```python
from build123d import *

# Parameters (mm, degrees)
BOSS_EXTRUDE1_DEPTH      = 49
BOSS_EXTRUDE1_DEPTH_BACK = 49
BOSS_EXTRUDE2_DEPTH      = 5
BOSS_EXTRUDE4_DEPTH      = 15
BOSS_EXTRUDE5_DEPTH      = 22
BOSS_EXTRUDE5_DEPTH_BACK = 22
BOSS_EXTRUDE6_REACH      = 127.363
SKETCH7_R                = 1.75
CUT_EXTRUDE1_DEPTH       = 25
SKETCH8_R                = 2.75
CUT_EXTRUDE2_DEPTH       = 25
FILLET1_R                = 10
FILLET2_R                = 3
SKETCH9_W                = 3
SKETCH9_H                = 102
BOSS_EXTRUDE7_DEPTH      = 25


with BuildPart() as part:
    # Sketch1 → Boss-Extrude1 (new, two sides: drawn at the far end of the back side and taken through both)
    with BuildSketch(Plane.XY.offset(-BOSS_EXTRUDE1_DEPTH_BACK)):
        Polygon((0, 0), (50, 40), (50, 20.790627288), (9.370425713, -11.713032142), (13.118595999, -16.398244998), (56, 17.906878203), (56, 52.483749085), (-3.748170285, 4.685212857), align=None)
    extrude(amount=BOSS_EXTRUDE1_DEPTH + BOSS_EXTRUDE1_DEPTH_BACK)

    # Sketch2 → Boss-Extrude2 (add)
    with BuildSketch(Plane.XY.offset(49)):
        Polygon((-3.748170285, 4.685212857), (13.118595999, -16.398244998), (56, 17.906878203), (56, 52.483749085), align=None)
    boss_extrude2 = extrude(amount=BOSS_EXTRUDE2_DEPTH)

    # Mirror1: Boss-Extrude2 across plane
    add(boss_extrude2.mirror(Plane.XY))

    # Sketch4 → Boss-Extrude4 (add)
    with BuildSketch(Plane(origin=(9.370425713, -11.713032142, 0), x_dir=(0.7808688094430303, 0.6246950475544244, 0), z_dir=(-0.6246950475544244, 0.7808688094430304, 0))):
        Polygon((52.031242374, 49), (0, 49), (52.031242374, 44), align=None)
        Polygon((52.031242374, -49), (52.031242374, -44), (0, -49), align=None)
    extrude(amount=BOSS_EXTRUDE4_DEPTH)

    # Sketch5 → Boss-Extrude5 (add, two sides: drawn at the far end of the back side and taken through both)
    with BuildSketch(Plane(origin=(56, 0, 0), x_dir=(0, 0, -1), z_dir=(1, 0, 0)).offset(-BOSS_EXTRUDE5_DEPTH_BACK)):
        with BuildLine():
            Line((-49, 101.483749085), (-59, 101.483749085))
            Line((-59, 101.483749085), (-59, 98.483749085))
            Line((-59, 98.483749085), (-51.91338941, 98.483749085))
            ThreePointArc((-51.91338941, 98.483749085), (0, 49.483749085), (51.91338941, 98.483749085))
            Line((51.91338941, 98.483749085), (59, 98.483749085))
            Line((59, 98.483749085), (59, 101.483749085))
            Line((59, 101.483749085), (49, 101.483749085))
            ThreePointArc((49, 101.483749085), (0, 52.483749085), (-49, 101.483749085))
        make_face()
    extrude(amount=BOSS_EXTRUDE5_DEPTH + BOSS_EXTRUDE5_DEPTH_BACK)

    # Boss-Extrude6: up to this face of the body (flat: up to its plane)
    boss_extrude6_end = Plane(part.part.faces().sort_by_distance((25.735702215, 28.272310857, 0))[0])
    # Sketch6 → Boss-Extrude6 (add, up to the picked face)
    with BuildSketch(Plane.ZY.offset(-34), mode=Mode.PRIVATE) as boss_extrude6_sk1:
        with BuildLine():
            Line((-35, 63.025980039), (-35, 33.025980039))
            Line((-35, 33.025980039), (35, 33.025980039))
            Line((35, 33.025980039), (35, 63.025980039))
            ThreePointArc((35, 63.025980039), (0, 49.483749085), (-35, 63.025980039))
        make_face()
    boss_extrude6_tool1 = split(extrude(boss_extrude6_sk1.sketch, amount=-BOSS_EXTRUDE6_REACH, mode=Mode.PRIVATE), bisect_by=boss_extrude6_end, keep=Keep.BOTH, mode=Mode.PRIVATE)
    add(boss_extrude6_tool1.solids().sort_by(Axis((34, 43.754603, 0), (1, 0, 0)))[0])

    # Sketch7 → Cut-Extrude1 (cut)
    with BuildSketch(Plane(origin=(0, 101.483749085, 0), x_dir=(1, 0, 0), z_dir=(0, 1, 0))):
        with Locations(Location((56, 53.5, 0), (0, 0, 270))):
            Circle(SKETCH7_R)
        with Locations(Location((41, 53.5, 0), (0, 0, 270))):
            Circle(SKETCH7_R)
        with Locations(Location((71, 53.5, 0), (0, 0, 270))):
            Circle(SKETCH7_R)
        with Locations(Location((71, -53.5, 0), (0, 0, 65.044347067))):
            Circle(SKETCH7_R)
        with Locations(Location((56, -53.5, 0), (0, 0, 65.044347067))):
            Circle(SKETCH7_R)
        with Locations(Location((41, -53.5, 0), (0, 0, 65.044347067))):
            Circle(SKETCH7_R)
    extrude(amount=-CUT_EXTRUDE1_DEPTH, mode=Mode.SUBTRACT)

    # Sketch8 → Cut-Extrude2 (cut)
    with BuildSketch(Plane.XZ.offset(-98.483749085)):
        with Locations((41, -53.5)):
            Circle(SKETCH8_R)
        with Locations((56, -53.5)):
            Circle(SKETCH8_R)
        with Locations((71, -53.5)):
            Circle(SKETCH8_R)
        with Locations((71, 53.5)):
            Circle(SKETCH8_R)
        with Locations((56, 53.5)):
            Circle(SKETCH8_R)
        with Locations((41, 53.5)):
            Circle(SKETCH8_R)
    extrude(amount=CUT_EXTRUDE2_DEPTH, mode=Mode.SUBTRACT)

    # Fillet1
    fillet1_edges = [part.edges().sort_by_distance(p)[0] for p in [
        (34, 48.954864562, 35),
        (34, 48.954864562, -35),
    ]]
    fillet(fillet1_edges, radius=FILLET1_R)

    # Fillet2
    fillet2_edges = [part.edges().sort_by_distance(p)[0] for p in [
        (56, 17.906878203, 0),
        (26.125914857, 28.584480971, 54),
        (34.559297999, 0.754316602, 54),
        (56, 35.195313644, 54),
        (26.125914857, 28.584480971, -54),
        (56, 35.195313644, -54),
        (34.559297999, 0.754316602, -54),
    ]]
    fillet(fillet2_edges, radius=FILLET2_R)

    # Sketch9 → Boss-Extrude7 (add)
    with BuildSketch(Plane(origin=(-3.748170285, 4.685212857, 0), x_dir=(0.7808688094430302, 0.6246950475544245, 0), z_dir=(-0.6246950475544245, 0.7808688094430302, 0))):
        with Locations((1.5, 0)):
            Rectangle(SKETCH9_W, SKETCH9_H)
    extrude(amount=BOSS_EXTRUDE7_DEPTH)


solid = part.part
```
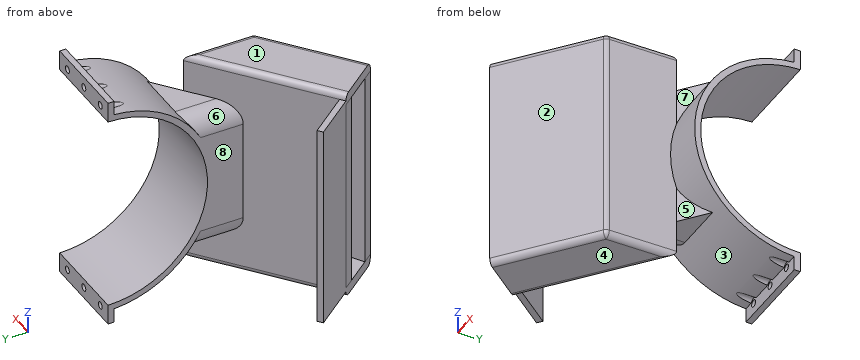
Work out the finished part from the listing and answer in its coordinate system (mm). Face numbers are marked on the shaded views. A direction names the side the tool comes from. Give positions to 0.01 mm unless a question says otherwise; leave off trailing zeros. Order: outer loops, then holes, each group sorted by start corner. A loop starts at its lowest first (then second) coordinate and runs counter-clockwise, first axis right, second up. Notation, with made-up numbers: M -37,6 L -27,6 A25 ccw -27,30 Z; hole C 32,87.5 d10. An arc over 180 degrees is marked long. Return JSON: item names as keys, results as strings.
1) For a pull along Y with two mould halves and no side action, classify the marked faces 1, 2 and 3 as +Y half, -Y half, draft (parallel to the pull), parting line (faces both ways), or undercut.
Resolved:
{"face 1": "draft", "face 2": "-Y half", "face 3": "undercut"}
2) Each of these flat-tipped pins is pushed along its axis until it touches: pin 1 (4.5 mm diameter, centred on x = 43.5, y = 27, fed in from +Z); pin 2 (16 mm diameter, centred on x = 57, y = 51.5, fed in from -Z); pin 3 (8 mm diameter, centred on y = 50, z = -42, fed in from -X); pin 4 (2 mm diameter, centred on x = 71, z = -53.5, fed in from +Y). Where does it stop, or does it pass through?
Resolved:
{"pin 1": "z = 54", "pin 2": "z = -54", "pin 3": "x = 47.9", "pin 4": "through"}
3) Section B-B, the plane y = 12 is taken. Give the number of separate pieces and of enclosed holes in the cut face, plus the area to 3 significant figures.
Resolved:
{"separate pieces": "2", "enclosed holes": "1", "area": "2,830 mm^2"}
4) Section A-A, the plane z = 37.5 is taken. Write down the section's boundary in (x, y), plus the area to 3 significant figures.
Resolved:
{"outline": "M -19.37,24.21 L 0,0 L 50,40 L 50,20.79 L 9.37,-11.71 L 13.12,-16.4 L 54.87,17.01 A3 ccw 56,19.35 L 56,52.48 L -1.41,6.56 L -17.02,26.08 Z; M 34,65.46 L 78,65.46 L 78,69.94 L 34,69.94 Z", "area": "1,180 mm^2"}
5) Straight lines are drawn through the part: line 1 along X through (y, z) = (99.85, 53.5); line 2 along Y through (x, z) = (20, -17); line 3 along Z through (x, y) = (46.5, 67). For each, find the intervals that lie inside material, in ascending order. Write a range as [from, to].
Resolved:
{"line 1": "[34, 39.25], [42.75, 54.25], [57.75, 69.25], [72.75, 78]", "line 2": "[-10.89, -3.21], [16, 23.68]", "line 3": "[-38.92, -34.81], [34.81, 38.92]"}
6) A tool of negligible diameter and unlimited length cuts with its end or side. For the marked faces 4, 5, 6, 7 and 8, from which of +Z, -Z, +X, -X, +Y, -Y can it reach the whole face along a straight path? Write none if from no direction.
Resolved:
{"face 4": "-Z, +X, -X, -Y", "face 5": "-Z, +X, -Y", "face 6": "+Z, -X", "face 7": "+Z, +X, -Y", "face 8": "+Z, -Z, -X, +Y"}
7) Section C-C, the plane z = 23 is taken. Write down the section's boundary in (x, y).
Resolved:
{"outline": "M -19.37,24.21 L 0,0 L 50,40 L 50,20.79 L 9.37,-11.71 L 13.12,-16.4 L 54.87,17.01 A3 ccw 56,19.35 L 56,52.48 L 58.95,54.85 L 78,54.85 L 78,58.22 L 34,58.22 L 34,34.88 L -1.41,6.56 L -17.02,26.08 Z"}
